Solid Edge part; units mm, degrees
sketch "Sketch1" plane through (0, 0, 0) normal (0, 0, 1) x (1, 0, 0)
  circle A0 centre (0, 0) radius 2.413
extrude "Protrusion1" add sketch "Sketch1" along normal blind 19.05
chamfer "Chamfer1" distance 0.3619 angle 45 2 edges at (-2.413, 0, 0) (-2.413, 0, 19.05)
sketch "Sketch2" plane through (0, 0, 19.05) normal (0, 0, 1) x (1, 0, 0)
  line L0 (-0.6878, 1.1913) -> (0.6878, 1.1913)
  line L1 (1.3755, 0) -> (0.6878, 1.1913)
  line L2 (0.6878, -1.1913) -> (1.3755, 0)
  line L3 (-0.6878, -1.1913) -> (0.6878, -1.1913)
  line L4 (-1.3755, 0) -> (-0.6878, -1.1913)
  line L5 (-0.6878, 1.1913) -> (-1.3755, 0)
extrude "Cutout1" cut sketch "Sketch2" against normal blind 9.525
properties part number "24101738"
Input: part model. Units: mm. Frame: model coordinates. A direction names the side the tool comes from. Give positions to 0.01 mm unless a question says otherwise; leave off trailing zeros. Write each loop counter-clockwise with the first axis right and the second up, starting at its lowest first coordinate (ties: lowest second). Pieces come first, ordered by that corner, then holes. Notation, with made-up numbers: (23.5, 37.5) -> (41.5, 37.5) arc R17 ccw to (41.5, 48.5) -> close; hole circle Ø5 at (38, -18). An arc over 180 degrees is marked (long way). Use one line per item in the form item = value. Start each with the question number.
1) Section query B-B on x = 0. Return the cut outline in (y, z) (3 decimals).
2) Pin query (flat end, axial travel): pin 1 (1.5 mm diameter, centred on x = 1, z = 10, fed in from +Y). Return the tip coordinate at first contact, or that it passes through.
3) Draft query along X for faces 3 (the flat face through (1, -1, 19.05)), 4 (the flat face through (0, 1.191, 14)), 5 (the cylindrical face through (-1.915, 1.468, 9.397)). Return one class per face: pulls with the +X half, pulls with the -X half, needs draft (parallel to the pull), parting line crosses it, or undercut.
4) Section query C-C on z = 6.25. Return the cut outline in (x, y).
5) Set-up query: faces 1 (the flat face through (0, 0, 0)), 2 (the flat face through (0, -1.191, 14)). Return all of +Z, -Z, +X, -X, +Y, -Y with unobstructed straight access to the full face (end or side cutting, diameter ignored); none if empty.
6) Ray query, probe 1 along Z at (x, y) = (-0.6, 0.95) (3 decimals); probe 2 along X at (y, z) = (2.1, 17); probe 3 along X at (y, z) = (-1.05, 14.5). Return the intervals inside material, ascending. Write a range as from..to.
7) Section query A-A on z = 15.5. Return the cut outline in (x, y), then the cut area to 3 significant figures.
Outcome:
q1.outline = (-2.413, 0.362) -> (-2.051, 0) -> (2.051, 0) -> (2.413, 0.362) -> (2.413, 18.688) -> (2.051, 19.05) -> (1.191, 19.05) -> (1.191, 9.525) -> (-1.191, 9.525) -> (-1.191, 19.05) -> (-2.051, 19.05) -> (-2.413, 18.688) -> close
q2.pin_1 = 2.4
q3.face_3 = needs draft
q3.face_4 = undercut
q3.face_5 = parting line crosses it
q4.outline = circle Ø4.83 at (0, 0)
q5.face_1 = -Z, +X, -X, +Y, -Y
q5.face_2 = +Z
q6.probe_1 = 0..9.525
q6.probe_2 = -1.19..1.19
q6.probe_3 = -2.17..-0.77, 0.77..2.17
q7.outline = circle Ø4.83 at (0, 0); hole (-1.38, 0) -> (-0.69, -1.19) -> (0.69, -1.19) -> (1.38, 0) -> (0.69, 1.19) -> (-0.69, 1.19) -> close
q7.area = 13.4 mm^2
